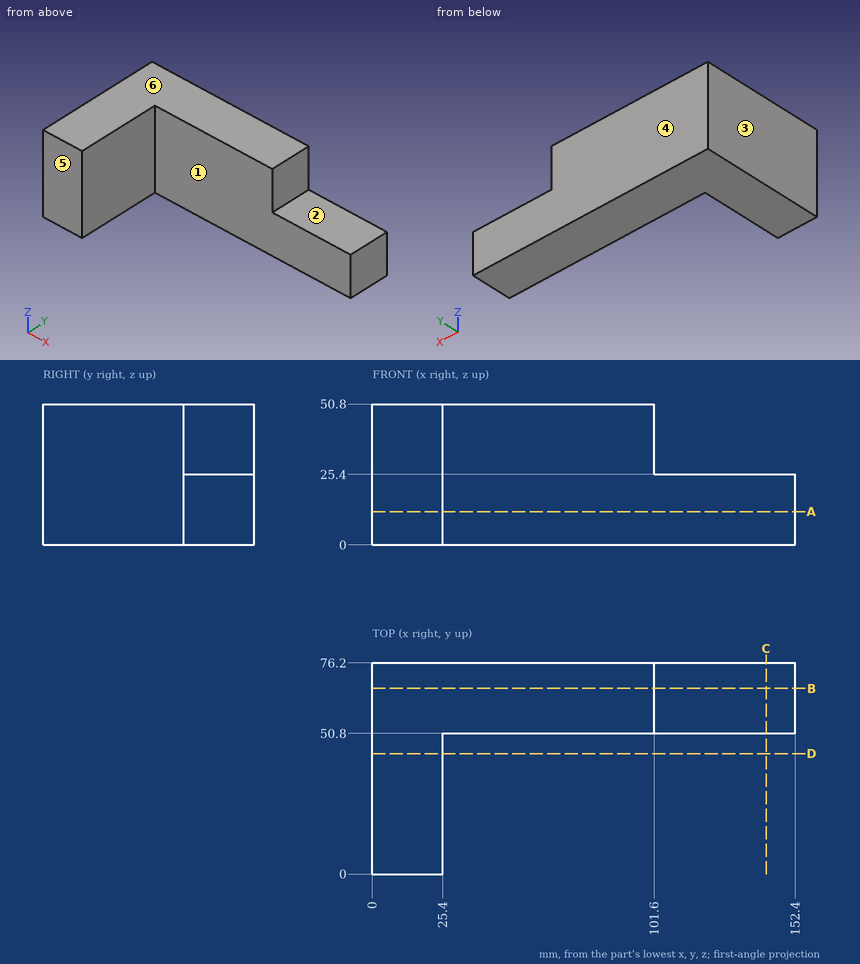
Study the drawing (mm; zero at the part's minimum x, y, z) and answer. A direction names the side the tool comes from. Coordinates: 2 decimals unless noted, no trailing zeros. Loops run counter-clockwise (first coordinate to the right, second up) from the corner with the lowest first, then second, coordinate; pieces in that order, holes last. Notation, with made-up numbers: (-5, -37.75) -> (3, -37.75) arc R20 ccw to (3, -2.75) -> close; hole circle Ø1 at (48.5, 32.25). An arc over 180 degrees is marked (long way). Write item = value, one per line. Start each with the question number.
1) The part is cut by section A-A, the plane z = 12. Determine the outline of the cut face in (x, y).
2) For the marked faces 1, 2 and 3, determine the directions among +Z, -Z, +X, -X, +Y, -Y from which every point of the face is accessible in a straight line to the end or side of a thin tool.
3) Given P1, Ø12, axis at x = 36, y = 52.5, coming from the -Z side; P2, Ø10, axis at y = 45.5, z = 15, coming from the +X side; P3, Ø20.5, axis at y = 62.5, z = 40.5, coming from the +X side; P4, Ø8, axis at x = 106, z = 27.5, coming from the -Y side, each flat-ended and moving along its own axis, determine where each tip first touches the part or whether it passes through.
4) The part is cut by section C-C, the plane x = 142. Determine the outline of the cut face in (y, z).
5) The mould has two halves that part along Y. Classify the marked faces 4, 5 and 6: pulls with the +Y half, pulls with the -Y half, needs draft (parallel to the pull), parting line crosses it, or undercut.
6) The part is cut by section B-B, the plane y = 67. Determine the outline of the cut face in (x, z).
7) The part is cut by section D-D, the plane y = 43.5. Determine the outline of the cut face in (x, z).
8) Find the intervals of material crossed by L1, parallel to X at y = 64, z = 38.5; L2, parallel to X at y = 24, z = 47.5; L3, parallel to Y at x = 66, z = 10, in increasing order. Write a range as from..to.
Result:
q1.outline = (0, 0) -> (25.4, 0) -> (25.4, 50.8) -> (152.4, 50.8) -> (152.4, 76.2) -> (0, 76.2) -> close
q2.face_1 = +Z, -Z, +X, -Y
q2.face_2 = +Z, +X, +Y, -Y
q2.face_3 = +Z, -Z, -X, +Y, -Y
q3.P1 = 0
q3.P2 = 25.4
q3.P3 = 101.6
q3.P4 = 50.8
q4.outline = (50.8, 0) -> (76.2, 0) -> (76.2, 25.4) -> (50.8, 25.4) -> close
q5.face_4 = pulls with the +Y half
q5.face_5 = pulls with the -Y half
q5.face_6 = needs draft
q6.outline = (0, 0) -> (152.4, 0) -> (152.4, 25.4) -> (101.6, 25.4) -> (101.6, 50.8) -> (0, 50.8) -> close
q7.outline = (0, 0) -> (25.4, 0) -> (25.4, 50.8) -> (0, 50.8) -> close
q8.L1 = 0..101.6
q8.L2 = 0..25.4
q8.L3 = 50.8..76.2
